For this review, take the finished solid that the model builds, in its own axes (mm). Face numbers are marked on the shaded views. A direction names the side the tool comes from. Round coordinates to 2 decimals unless told otherwise and drop trailing zeros. Write each loop counter-clockwise with the first axis right and the second up, starting at its lowest first coordinate (ties: lowest second). Pieces come first, ordered by that corner, then holes. Notation, with made-up numbers: M 41,-6 L 83,-6 A20 cw 83,-1 Z; hole C 69.5,55 d11. An arc over 180 degrees is marked long. One line per question, with ' | ' between items.
```python
from build123d import *

# Parameters (mm, degrees)
SKETCH1_W           = 101.6
SKETCH1_H           = 101.6
BOSS_EXTRUDE1_DEPTH = 127
SKETCH2_W           = 86.36
SKETCH2_H           = 86.36
CUT_EXTRUDE1_DEPTH  = 116.84
SKETCH4_W           = 20.32
SKETCH4_H           = 20.32
SKETCH4_W_2         = 15.24
SKETCH4_H_2         = 15.24
BOSS_EXTRUDE2_DEPTH = 17.78
SKETCH6_R           = 7.62
CUT_EXTRUDE2_DEPTH  = 1.27
SKETCH7_W           = 20.32
SKETCH7_H           = 20.32
SKETCH7_W_2         = 15.24
SKETCH7_H_2         = 15.24
BOSS_EXTRUDE3_DEPTH = 17.78
SKETCH9_R           = 7.62
CUT_EXTRUDE3_DEPTH  = 1.27
FILLET1_R           = 1.27


with BuildPart() as part:
    # Sketch1 → Boss-Extrude1 (new body)
    with BuildSketch(Plane.XY):
        Rectangle(SKETCH1_W, SKETCH1_H)
    extrude(amount=BOSS_EXTRUDE1_DEPTH)

    # Sketch2 → Cut-Extrude1 (cut)
    with BuildSketch(Plane.XY.offset(127)):
        Rectangle(SKETCH2_W, SKETCH2_H)
    extrude(amount=-CUT_EXTRUDE1_DEPTH, mode=Mode.SUBTRACT)

    # Sketch4 → Boss-Extrude2 (add)
    with BuildSketch(Plane(origin=(0, 50.8, 0), x_dir=(1, 0, 0), z_dir=(0, 1, 0))):
        with Locations((0, -63.5)):
            Rectangle(SKETCH4_W, SKETCH4_H)
        with Locations((0, -63.5)):
            Rectangle(SKETCH4_W_2, SKETCH4_H_2, mode=Mode.SUBTRACT)
    boss_extrude2 = extrude(amount=BOSS_EXTRUDE2_DEPTH)

    # Sketch6 → Cut-Extrude2 (cut)
    with BuildSketch(Plane(origin=(0, 50.8, 0), x_dir=(1, 0, 0), z_dir=(0, 1, 0))):
        with Locations(Location((0, -63.5, 0), (0, 0, 180))):
            Circle(SKETCH6_R)
    cut_extrude2 = extrude(amount=-CUT_EXTRUDE2_DEPTH, mode=Mode.SUBTRACT)

    # Mirror1: Boss-Extrude2, Cut-Extrude2 across plane
    add(boss_extrude2.mirror(Plane.ZX))
    add(cut_extrude2.mirror(Plane.ZX), mode=Mode.SUBTRACT)

    # Sketch7 → Boss-Extrude3 (add)
    with BuildSketch(Plane(origin=(50.8, 0, 0), x_dir=(0, 0, -1), z_dir=(1, 0, 0))):
        with Locations((-63.5, 0)):
            Rectangle(SKETCH7_W, SKETCH7_H)
        with Locations((-63.5, 0)):
            Rectangle(SKETCH7_W_2, SKETCH7_H_2, mode=Mode.SUBTRACT)
    boss_extrude3 = extrude(amount=BOSS_EXTRUDE3_DEPTH)

    # Sketch9 → Cut-Extrude3 (cut)
    with BuildSketch(Plane(origin=(50.8, 0, 0), x_dir=(0, 0, -1), z_dir=(1, 0, 0))):
        with Locations((-63.5, 0)):
            Circle(SKETCH9_R)
    cut_extrude3 = extrude(amount=-CUT_EXTRUDE3_DEPTH, mode=Mode.SUBTRACT)

    # Mirror2: Boss-Extrude3, Cut-Extrude3 across plane
    add(boss_extrude3.mirror(Plane(origin=(0, 0, 0), x_dir=(0, 0, 1), z_dir=(1, 0, 0))))
    add(cut_extrude3.mirror(Plane(origin=(0, 0, 0), x_dir=(0, 0, 1), z_dir=(1, 0, 0))), mode=Mode.SUBTRACT)

    # Fillet1
    fillet1_edges = [part.edges().sort_by_distance(p)[0] for p in [
        (50.8, 0, 127),
        (0, 50.8, 127),
        (-50.8, 0, 127),
        (0, 50.8, 0),
        (50.8, 0, 0),
        (0, -50.8, 0),
        (-50.8, 0, 0),
        (0, -50.8, 127),
        (-50.8, 50.8, 63.5),
        (50.8, 50.8, 63.5),
        (50.8, -50.8, 63.5),
        (-50.8, -50.8, 63.5),
    ]]
    fillet(fillet1_edges, radius=FILLET1_R)


solid = part.part
```
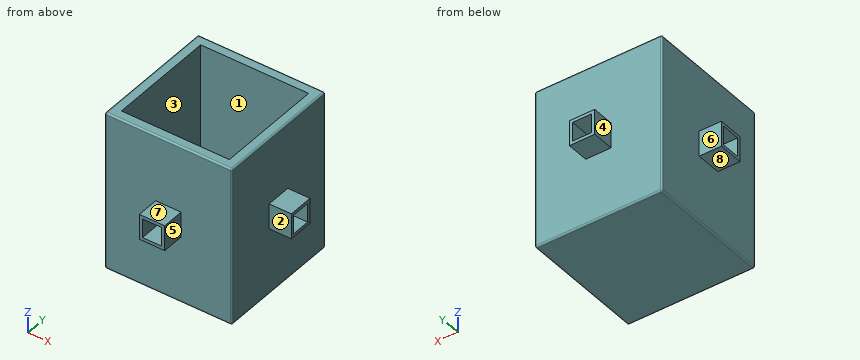
Item 1: Machinability: for the marked faces 5, 6, 7 and 8, which of the approach directions +Z, -Z, +X, -X, +Y, -Y give a long, thin tool a straight path to every point of the face, cutting with its end or side? Answer none if there is none.
Results:
face 5: +Z, -Z, +X, -Y | face 6: +Z, -Z, -X, +Y | face 7: +Z, +X, -X, -Y | face 8: -Z, -X, +Y, -Y
Item 2: To check wall thickness, follow line 1 along Z through (x, y) = (-54, -2.5); line 2 along Y through (x, z) = (-10, 61.5); line 3 along X through (y, z) = (23, 35). State the ranges of each line that lie inside material, in increasing order. Write a range as from..to.
Results:
line 1: 53.34..55.88, 71.12..73.66 | line 2: -68.58..-43.18, 43.18..68.58 | line 3: -50.8..-43.18, 43.18..50.8
Item 3: Take a section at D-D (x = -21.5). Write out the cut boundary in (y, z), then the cut area to 3 significant figures.
Results:
outline: M -50.8,1.27 A1.27 ccw -49.53,0 L 49.53,0 A1.27 ccw 50.8,1.27 L 50.8,125.73 A1.27 ccw 49.53,127 L 43.18,127 L 43.18,10.16 L -43.18,10.16 L -43.18,127 L -49.53,127 A1.27 ccw -50.8,125.73 Z | area: 2,810 mm2
Item 4: Take a section at B-B (z = 85.5). Write out the cut boundary in (x, y), then the cut area to 3 significant figures.
Results:
outline: M -50.8,-49.53 A1.27 ccw -49.53,-50.8 L 49.53,-50.8 A1.27 ccw 50.8,-49.53 L 50.8,49.53 A1.27 ccw 49.53,50.8 L -49.53,50.8 A1.27 ccw -50.8,49.53 Z; hole M -43.18,-43.18 L 43.18,-43.18 L 43.18,43.18 L -43.18,43.18 Z | area: 2,860 mm2
Item 5: Take a section at A-A (x = 53.5). Write out the cut boundary in (y, z).
Results:
outline: M -10.16,53.34 L 10.16,53.34 L 10.16,73.66 L -10.16,73.66 Z; hole M -7.62,55.88 L 7.62,55.88 L 7.62,71.12 L -7.62,71.12 Z
Item 6: Mouldability with a two-part tool opening along X and no side actions: class the marked faces 1, 2, 3 and 4 as +X half, -X half, draft (parallel to the pull), parting line (faces both ways), or undercut.
Results:
face 1: undercut | face 2: draft | face 3: undercut | face 4: -X half
Item 7: Insertion check: pin 1 Ø6 at (x, z) = (4.5, 67) entering from +Y; pin 2 Ø6 at (x, z) = (3, 61) entering from -Y; pin 3 Ø14 at (x, z) = (62.5, 59.5) entering from +Y. Each pin has a flat end and moves straight along its axis. Give the tip position at first contact, or say it passes through.
Results:
pin 1: y = 50.8 | pin 2: y = -49.53 | pin 3: y = 10.16
